For this review, take the finished solid that the model builds, in its own axes (mm). Face numbers are marked on the shaded views. Round coordinates to 2 decimals unless told otherwise and drop trailing zeros. Loops run counter-clockwise (first coordinate to the right, second up) from the corner with the lowest first, then second, coordinate; pieces in that order, holes last.
1. Draft analysis for pull direction Z (two halves, no side actions). For the marked faces 1, 2 and 3, state which applies: released by +Z, released by -Z, zero draft, split by the parting line, or undercut.
2. To check wall thickness, follow line 1 along Y through (x, z) = (0.5, 2.75); line 2 along Y through (x, z) = (-0.25, 3.5); line 3 along Z through (x, y) = (0, 11). State the ranges of each line that lie inside material, in increasing order.
3. Clearance check with flat-ended pins moving along their axes: pin 1 Ø1 at (x, y) = (0, 11.5) entering from +Z; pin 2 Ø2.5 at (x, z) = (0, 0) entering from -Y; pin 3 Ø1 at (y, z) = (2.5, 2) entering from -X; pin 4 Ø3 at (x, z) = (-2.5, 2) entering from +Y. State where each tip first meets the part, or that it passes through.
4. Consider section A-A on y = 5. State the section outline as (x, z) points, then the cut area to 3 significant figures.
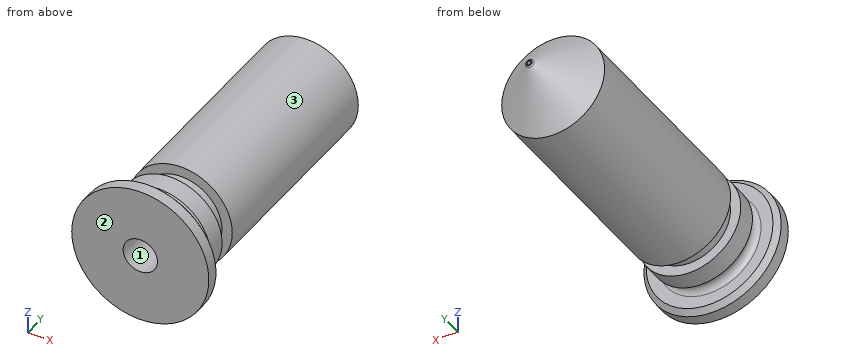
Autodesk Inventor part; units mm, degrees
ref_plane "XZ Plane" through (0, 0, 0) normal (0, 1, 0) x (-1, 0, 0)
sketch "Sketch1" plane through (0, 0, 0) normal (0, 1, 0) x (-1, 0, 0)
  circle A0 centre (0, 0) radius 4
  dimension "d0" = 8
extrude "Extrusion1" add sketch "Sketch1" along normal blind 1
sketch "Sketch2" plane through (0, 1, 0) normal (0, 1, 0) x (1, 0, 0)
  circle A0 centre (0, 0) radius 4
  circle A1 centre (0, 0) radius 3
  dimension "d3" = 6
extrude "Extrusion2" add sketch "Sketch2" along normal blind 15.437 contours A1
sketch "Sketch3" plane through (0, 0, 0) normal (0, -1, 0) x (1, 0, 0)
  circle A0 centre (0, 0) radius 4
  circle A1 centre (0, 0) radius 1
  dimension "d6" = 2
extrude "Extrusion3" cut sketch "Sketch3" against normal blind 21 contours A1
sketch "Sketch4" plane through (0, 0, 0) normal (1, 0, 0) x (0, 1, 0)
  line L0 (1, 3) -> (16.437, 3)
  line L1 (1, -3) -> (16.437, -3)
  line L2 (0, 0) -> (17, 0)
  line L3 (16.437, 3) -> (18.7445, 0.25)
  line L4 (16.437, -3) -> (16.437, 3)
  line L5 (16.437, 0.2) -> (17.8226, 0.2)
  line L6 (17.8226, 0.2) -> (16.437, 1)
  line L7 (0, 1) -> (16.437, 1)
  line L8 (16.437, 1) -> (16.437, 3)
  line L9 (17.9525, 0.125) -> (18.8075, 0.125)
  line L10 (17.8226, 0.2) -> (17.9525, 0.125)
  line L11 (18.7445, 0.25) -> (18.8075, 0.175)
  line L12 (18.8075, 0.125) -> (18.8075, 0.175)
  dimension "d9" = 40
  dimension "d10" = 0.2
  dimension "d11" = 30
  dimension "d21" = 0.125
  dimension "d22" = 0.05
revolve "Revolution1" add sketch "Sketch4" angle 360 about axis through (0, 0, 0) along (0, 1, 0) contours L3 L11 L12 L9 L10 L6 L4
sketch "Sketch5" plane through (0, 0, 0) normal (0, 0, 1) x (1, 0, 0)
  circle A0 centre (3, 1.35) radius 0.35
  line L0 (4, 1) -> (-4, 1)
  line L1 (3, 3) -> (3, 0)
  line L2 (0, 1.1204) -> (0, 3)
  line L3 (2.7525, 1.5975) -> (3.3734, 2.2184)
  line L4 (3.3734, 2.2184) -> (3.3499, 1.3406)
  point P0 (0, 0)
  dimension "d14" = 0.7
  dimension "d19" = 45
revolve "Revolution2" cut sketch "Sketch5" angle 360 about axis through (0, 1.1204, 0) along (0, 1, 0)
chamfer "Chamfer1" distance 0.3 angle 45 1 edges at (4, 1, 0)
sketch "Sketch6" plane through (0, 0, 0) normal (1, 0, 0) x (0, 1, 0)
  line L0 (1.845, -3) -> (16.437, -3)
  line L1 (3, -3) -> (4, -3)
  line L2 (4, -3) -> (4, -2.4)
  line L3 (4, -2.4) -> (3, -2.4)
  line L4 (3, -2.4) -> (3, -3)
  line L5 (0, 4) -> (0, -4)
  line L6 (0, 0) -> (-1.7649, 0)
  dimension "d23" = 1
  dimension "d24" = 0.6
  dimension "d25" = 3
revolve "Revolution3" cut sketch "Sketch6" angle 360 about axis through (0, 0, 0) along (0, -1, 0)
properties part number "nozzle0.25" material "Copper"
Resolved:
1. face 1: undercut
1. face 2: zero draft
1. face 3: split by the parting line
2. line 1: y = 0 to 1.07, 1.64 to 3, 4 to 16.61
2. line 2: y = 0 to 1
2. line 3: z = -3 to -1, 1 to 3
3. pin 1: stops at z = 3
3. pin 2: stops at y = 0
3. pin 3: stops at x = -2.6
3. pin 4: stops at y = 17.53
4. outline: circle Ø6 at (0, 0); hole circle Ø2 at (0, 0)
4. area: 25.1 mm2
